```python
from build123d import *

# Parameters (mm, degrees)
F0_W      = 9
F0_H      = 3.5
F1_DEPTH  = 11.2
F3_D      = 2.38
F3_DEPTH  = 3.25
F3_TIP    = 0.7150241366
F5_D      = 1.3
F6_W      = 9
F6_H      = 1
F7_DEPTH  = 0.3
F9_DEPTH  = 3.25
F10_W     = 9
F10_H     = 1
F11_DEPTH = 0.3


with BuildPart() as f1:
    # F0 (on Top) → F1 (new body)
    with BuildSketch(Plane.XY):
        Rectangle(F0_W, F0_H)
    extrude(amount=F1_DEPTH)

    # F3
    with Locations(Plane.XY.offset(11.2)):
        with Locations((0, 0)):
            Hole(F3_D / 2, depth=F3_DEPTH)
            with Locations((0, 0, -(F3_DEPTH + F3_TIP / 2))):  # 118° drill point
                Cone(0, F3_D / 2, F3_TIP, mode=Mode.SUBTRACT)

    # F5 (through all)
    with Locations(Plane.XY.offset(11.2)):
        with Locations((0, 0), (-2.85, 0), (2.85, 0)):
            Hole(F5_D / 2)

    # F6 (on face) → F7 (cut)
    with BuildSketch(Plane.XZ.offset(1.75)):
        with Locations((0, 2.3625027388)):
            Rectangle(F6_W, F6_H)
    extrude(amount=-F7_DEPTH, mode=Mode.SUBTRACT)

    # F8 (on face) → F9 (cut)
    with BuildSketch(Plane.XY.offset(11.2)):
        with BuildLine():
            Line((-1, -1.75), (1, -1.75))
            Line((1, -1.75), (1, -0.6450581369))
            ThreePointArc((1, -0.6450581369), (0, -1.19), (-1, -0.6450581369))
            Line((-1, -0.6450581369), (-1, -1.75))
        make_face()
        with BuildLine():
            ThreePointArc((-1, 0.6450581369), (0, 1.19), (1, 0.6450581369))
            Line((1, 0.6450581369), (1, 1.75))
            Line((1, 1.75), (-1, 1.75))
            Line((-1, 1.75), (-1, 0.6450581369))
        make_face()
    extrude(amount=-F9_DEPTH, mode=Mode.SUBTRACT)

    # F10 (on face) → F11 (cut)
    with BuildSketch(Plane(origin=(0, 1.75, 0), x_dir=(-1, 0, 0), z_dir=(0, 1, 0))):
        with Locations((0, 3.3379399683)):
            Rectangle(F10_W, F10_H)
    extrude(amount=-F11_DEPTH, mode=Mode.SUBTRACT)


solid = f1.part
```
Design review of the part built by this model. Coordinates are the model's own, in mm. A direction names the side the tool comes from. Coordinates: 2 decimals unless noted, no trailing zeros. Write each loop counter-clockwise with the first axis right and the second up, starting at its lowest first coordinate (ties: lowest second). Pieces come first, ordered by that corner, then holes. Notation, with made-up numbers: M 81.25,48 L 119.25,48 A7 ccw 119.25,58 Z; hole C 45,47.25 d9. An arc over 180 degrees is marked long. Answer as a JSON object with one key per item and string values.
Item 1: Wall thickness on probe 1 along Z at (x, y) = (1.25, 1.5); probe 2 along Z at (x, y) = (-0.75, -1.5); probe 3 along X at (y, z) = (0.9, 8.25): over which ranges is each line inside the solid? List them lowest first.
Outcome:
{"probe 1": "0 to 2.84, 3.84 to 11.2", "probe 2": "0 to 1.86, 2.86 to 7.95", "probe 3": "-4.5 to -1, 1 to 4.5"}
Item 2: Add section C-C, the plane y = 0. Give the boundary of the cut face in (x, z), and give its area (3 significant figures).
Outcome:
{"outline": "M -4.5,0 L -3.5,0 L -3.5,11.2 L -4.5,11.2 Z; M -2.2,0 L -0.65,0 L -0.65,7.63 L -1.19,7.95 L -1.19,11.2 L -2.2,11.2 Z; M 0.65,0 L 2.2,0 L 2.2,11.2 L 1.19,11.2 L 1.19,7.95 L 0.65,7.63 Z; M 3.5,0 L 4.5,0 L 4.5,11.2 L 3.5,11.2 Z", "area": "53.4 mm²"}
Item 3: Add section A-A, the plane z = 9.25. Give the boundary of the cut face in (x, y).
Outcome:
{"outline": "M -4.5,-1.75 L -1,-1.75 L -1,-0.65 A1.19 cw -1,0.65 L -1,1.75 L -4.5,1.75 Z; M 1,-1.75 L 4.5,-1.75 L 4.5,1.75 L 1,1.75 L 1,0.65 A1.19 cw 1,-0.65 Z; hole C -2.85,0 d1.3; hole C 2.85,0 d1.3"}
Item 4: Draft analysis for pull direction Y (two halves, no side actions). For faces 4 (the cylindrical face through (3.33, 0.44, 5.52)), 5 (the flat face through (-0.1, -1.45, 2.4)), 6 (the flat face through (-1, -1, 10)), state which applies: pulls with the +Y half, pulls with the -Y half, needs draft (parallel to the pull), parting line crosses it, or undercut.
Outcome:
{"face 4": "undercut", "face 5": "pulls with the -Y half", "face 6": "needs draft"}
Item 5: Add section B-B, the plane x = 0. Give the boundary of the cut face in (y, z), and give its area (3 significant figures).
Outcome:
{"outline": "M -1.75,0 L -0.65,0 L -0.65,7.63 L -1.19,7.95 L -1.75,7.95 L -1.75,2.86 L -1.45,2.86 L -1.45,1.86 L -1.75,1.86 Z; M 0.65,0 L 1.75,0 L 1.75,2.84 L 1.45,2.84 L 1.45,3.84 L 1.75,3.84 L 1.75,7.95 L 1.19,7.95 L 0.65,7.63 Z", "area": "16.7 mm²"}
Item 6: Add section D-D, the plane z = 2. Give the boundary of the cut face in (x, y), and give its area (3 significant figures).
Outcome:
{"outline": "M -4.5,-1.45 L 4.5,-1.45 L 4.5,1.75 L -4.5,1.75 Z; hole C -2.85,0 d1.3; hole C 0,0 d1.3; hole C 2.85,0 d1.3", "area": "24.8 mm²"}
Item 7: Insertion check: pin 1 Ø1 at (x, y) = (0, -1) entering from -Z; pin 2 Ø0.9 at (x, y) = (-0.5, -1) entering from +Z; pin 3 Ø2 at (x, y) = (0, 0) entering from +Z. Each pin has a flat end and moves straight along its axis. Give the tip position at first contact, or say it passes through.
Outcome:
{"pin 1": "z = 0", "pin 2": "z = 7.95", "pin 3": "z = 7.84"}
Item 8: Machinability: for faces 1 (the flat face through (0, -1.4, 7.95)), 2 (the cylindrical face through (1.19, 0.01, 9.55)), 3 (the flat face through (0, 1.45, 3)), which of the approach directions +Z, -Z, +X, -X, +Y, -Y give a long, thin tool a straight path to every point of the face, cutting with its end or side? Answer none if there is none.
Outcome:
{"face 1": "+Z, +Y, -Y", "face 2": "+Z", "face 3": "+X, -X, +Y"}
